```python
from build123d import *

# Parameters (mm, degrees)
SKETCH006_R      = 1.8
EXTRUDE004_DEPTH = 1
EXTRUDE005_DEPTH = 2
SKETCH017_R      = 3.8
SKETCH017_R_2    = 1.8
EXTRUDE014_DEPTH = 1
EXTRUDE003_DEPTH = 27.5


with BuildPart() as extrude004:
    # Sketch006 → Extrude004 (new body)
    with BuildSketch(Plane.XY.offset(10)):
        Polygon((-11, 0), (0, 0), (0, 12), (-23, 12), (-23, -21.5), (-11, -21.5), align=None)
        with Locations((-17, 6)):
            Circle(SKETCH006_R, mode=Mode.SUBTRACT)
    extrude(amount=EXTRUDE004_DEPTH)


with BuildPart() as extrude004_1:
    # Extrude004 placement: moved
    add(extrude004.part.moved(Location((0, 0, -36.5))))


with BuildPart() as extrude005:
    # Sketch007 → Extrude005 (new body)
    with BuildSketch(Plane.XY.offset(10)):
        Polygon((0, 12), (-23, 12), (-23, -21.5), (-22, -21.5), (-22, -2.25), (-13, -2.25), (-13, -21.5), (-11, -21.5), (-11, 0), (0, 0), (0, 1), (-22, 1), (-22, 11), (0, 11), align=None)
    extrude(amount=EXTRUDE005_DEPTH)


with BuildPart() as extrude005_1:
    # Extrude005 placement: moved
    add(extrude005.part.moved(Location((0, 0, -35.5))))


with BuildPart() as extrude014:
    # Sketch017 → Extrude014 (new body)
    with BuildSketch(Plane.XY.offset(10)):
        with Locations((-17, 6)):
            Circle(SKETCH017_R)
        with Locations((-17, 6)):
            Circle(SKETCH017_R_2, mode=Mode.SUBTRACT)
    extrude(amount=EXTRUDE014_DEPTH)


with BuildPart() as extrude014_1:
    # Extrude014 placement: moved
    add(extrude014.part.moved(Location((0, 0, -35.5))))


with BuildPart() as body006:
    # Sketch003 → Extrude003 (new body)
    with BuildSketch(Plane.XY):
        Polygon((-21, -0.25), (-11, -0.25), (-11, -21.5), (-12, -21.5), (-12, -1.25), (-21, -1.25), align=None)
    extrude(amount=-EXTRUDE003_DEPTH)


with BuildPart() as body006_1:
    # Extrude003 placement: moved
    add(body006.part.moved(Location((0, 0, 2))))

    # Fusion013: union Extrude004, Extrude005, Extrude014
    add(extrude004_1.part)
    add(extrude005_1.part)
    add(extrude014_1.part)


with BuildPart() as part_mirroring007:
    # Part__Mirroring007: instance of Body006
    add(body006_1.part.mirror(Plane(origin=(0, -21.5, 0), x_dir=(1, 0, 0), z_dir=(0, 1, 0))))


solid = part_mirroring007.part
```
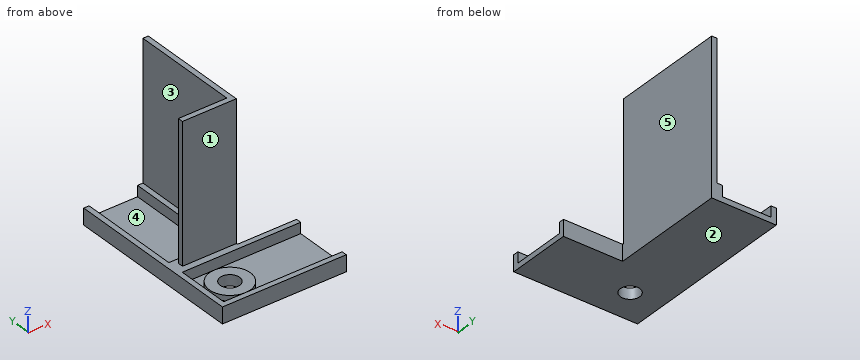
Work out the finished part from the listing and answer in its coordinate system (mm). Face numbers are marked on the shaded views. A direction names the side the tool comes from. Give positions to 0.01 mm unless a question says otherwise; leave off trailing zeros. Loops run counter-clockwise (first coordinate to the right, second up) from the corner with the lowest first, then second, coordinate; pieces in that order, holes last. Notation, with made-up numbers: (65, -16.5) -> (86, -16.5) arc R26 ccw to (86, 22.5) -> close; hole circle Ø2 at (1.5, -2). An arc over 180 degrees is marked (long way). One line per question, with ' | ' between items. Start each with the question number.
1) Section B-B, the plane x = -17 is taken. Determine the outline of the cut face in (y, z), then the cut area to 3 significant figures.
2) Determine the mould class of the marked faces 3, 4 and 5 for opening direction X: +X half, -X half, draft (parallel to the pull), parting line (faces both ways), or undercut.
3) Section D-D, the plane x = -8.5 is taken. Determine the outline of the cut face in (y, z).
4) Straight lines are drawn through the part: L1, parallel to Y at x = -21, z = -24.75; L2, parallel to X at y = -49, z = -25.85; L3, parallel to Y at x = -17, z = -25.55. For each, find the intervals that lie inside material, in ascending order.
5) Each of these flat-tipped pins is pushed along its axis until it touches: pin 1 (0.8 mm diameter, centred on y = -42.5, z = -9, fed in from -X); pin 2 (10 mm diameter, centred on x = -17.5, y = -27, fed in from +Z); pin 3 (12 mm diameter, centred on y = -33, z = -1, fed in from +X); pin 4 (10 mm diameter, centred on x = -4, y = -27.5, fed in from -Z). Where does it stop, or does it pass through?
6) Section A-A, the plane y = -49 is taken. Determine the outline of the cut face in (x, z).
7) For the marked faces 1 and 2, determine the directions among +Z, -Z, +X, -X, +Y, -Y from which every point of the face is accessible in a straight line to the end or side of a thin tool.
8) Section C-C, the plane y = -37.5 is taken. Determine the outline of the cut face in (x, z), then the cut area to 3 significant figures.
Resolved:
1) outline: (-55, -26.5) -> (-50.8, -26.5) -> (-50.8, -24.5) -> (-52.8, -24.5) -> (-52.8, -25.5) -> (-54, -25.5) -> (-54, -23.5) -> (-55, -23.5) -> close; (-47.2, -26.5) -> (-21.5, -26.5) -> (-21.5, -25.5) -> (-40.75, -25.5) -> (-40.75, -23.5) -> (-41.75, -23.5) -> (-41.75, 2) -> (-42.75, 2) -> (-42.75, -23.5) -> (-44, -23.5) -> (-44, -25.5) -> (-45.2, -25.5) -> (-45.2, -24.5) -> (-47.2, -24.5) -> close | area: 67.9 mm2
2) face 3: -X half | face 4: undercut | face 5: +X half
3) outline: (-55, -26.5) -> (-43, -26.5) -> (-43, -23.5) -> (-44, -23.5) -> (-44, -25.5) -> (-54, -25.5) -> (-54, -23.5) -> (-55, -23.5) -> close
4) L1: -55 to -54, -44 to -40.75 | L2: -23 to -18.8, -15.2 to 0 | L3: -55 to -50.8, -47.2 to -21.5
5) pin 1: x = -21 | pin 2: z = -23.5 | pin 3: x = -11 | pin 4: through
6) outline: (-23, -26.5) -> (-18.8, -26.5) -> (-18.8, -24.5) -> (-20.8, -24.5) -> (-20.8, -25.5) -> (-22, -25.5) -> (-22, -23.5) -> (-23, -23.5) -> close; (-15.2, -26.5) -> (0, -26.5) -> (0, -25.5) -> (-13.2, -25.5) -> (-13.2, -24.5) -> (-15.2, -24.5) -> close
7) face 1: +Z, +X, -X, -Y | face 2: -Z, +X, -X, +Y, -Y
8) outline: (-23, -26.5) -> (-11, -26.5) -> (-11, 2) -> (-12, 2) -> (-12, -23.5) -> (-13, -23.5) -> (-13, -25.5) -> (-22, -25.5) -> (-22, -23.5) -> (-23, -23.5) -> close | area: 43.5 mm2
